Verification items for the finished model (mm, model axes). A direction names the side the tool comes from. Coordinates: 2 decimals unless noted, no trailing zeros. Loops run counter-clockwise (first coordinate to the right, second up) from the corner with the lowest first, then second, coordinate; pieces in that order, holes last. Notation, with made-up numbers: (-35, 36) - (-8, 36) arc R21 ccw to (-8, 45) - close; hole circle Ø7 at (-33, -39.5). An arc over 180 degrees is marked (long way). One line per item, written item: value. Start each with the question number.
(1) Thickness scan on probe 1 along Y at (x, z) = (-50, 6); probe 2 along Y at (x, z) = (11, 66); probe 3 along Y at (x, z) = (-3.5, 134.5). Record the ranges inside material, lowest first. Write a range as [from, to].
(2) Gauge pin test, flat ends, axial feed: P1, Ø12, axis at y = 24.5, z = 31, coming from the -X side; P2, Ø5, axis at x = -6, y = 2.5, coming from the +Z side; P3, Ø6, axis at x = 33, y = -17.5, coming from the -Z side; P4, Ø4, axis at x = -12, z = 26, coming from the -Y side. Record the tip position at first contact, or that the pin passes through.
(3) Section check B-B (y = -20). Record the boundary of the cut face in (x, z).
(4) Draft check along Z on faces 4 (the face through (-58, -32, 10)), 5 (the face through (0, -18, 70)), 6 (the face through (32, 25, 21)). Enter one of: +Z half, -Z half, draft (parallel to the pull), parting line (faces both ways), or undercut.
(5) Set-up check for faces 1 (the face through (-6.503, -29.126, 149.287)), 2 (the face through (30, 26, 72)), 3 (the face through (4, 15, 129)): record each of +Z, -Z, +X, -X, +Y, -Y from which the full face is reachable in a straight line by a thin tool's end or side.
(6) Section check C-C (z = 132). Record the boundary of the cut face in (x, y), plus the area to 3 significant figures.
(7) Section check A-A (x = -50). Record the boundary of the cut face in (y, z).
(8) Section check D-D (x = 0). Record the boundary of the cut face in (y, z), plus the area to 3 significant figures.
```python
from build123d import *

# Parameters (mm, degrees)
Y_KSEKLIK_EKSTR_ZYON1_DEPTH = 20
Y_KSEKLIK_EKSTR_ZYON2_DEPTH = 15
Y_KSEKLIK_EKSTR_ZYON3_START = 3
IZIM3_R                     = 30
Y_KSEKLIK_EKSTR_ZYON3_DEPTH = 3
IZIM4_R                     = 20
Y_KSEKLIK_EKSTR_ZYON4_DEPTH = 3
IZIM5_R                     = 10
KES_EKSTR_ZYON1_DEPTH       = 169.534862862
AYNALAMA1_START             = -33
AYNALAMA1_OUTLINE_R         = 10
AYNALAMA1_DEPTH             = 15
AYNALAMA1_START_2           = -36
AYNALAMA1_2_OUTLINE_R       = 30
AYNALAMA1_2_OUTLINE_R_2     = 10
AYNALAMA1_2_DEPTH           = 3
AYNALAMA1_START_3           = -18
AYNALAMA1_3_OUTLINE_R       = 20
AYNALAMA1_3_OUTLINE_R_2     = 10
AYNALAMA1_3_DEPTH           = 3
IZIM6_R                     = 5.25
KES_EKSTR_ZYON2_DEPTH       = 148.634684272
RADYUS1_R                   = 5


# Read off the part's stored shape, not the designer's step: Aynalama1
with BuildPart() as part:
    # izim1 → Y_kseklik-Ekstr_zyon1 (new body)
    with BuildSketch(Plane.XY):
        with BuildLine():
            Line((-55, 33), (55, 33))
            ThreePointArc((55, 33), (58.535533906, 31.535533906), (60, 28))
            Line((60, 28), (60, -28))
            ThreePointArc((60, -28), (58.535533906, -31.535533906), (55, -33))
            Line((55, -33), (-55, -33))
            ThreePointArc((-55, -33), (-58.535533906, -31.535533906), (-60, -28))
            Line((-60, -28), (-60, 28))
            ThreePointArc((-60, 28), (-58.535533906, 31.535533906), (-55, 33))
        make_face()
    extrude(amount=Y_KSEKLIK_EKSTR_ZYON1_DEPTH)

    # izim2 → Y_kseklik-Ekstr_zyon2 (add)
    with BuildSketch(Plane(origin=(0, 33, 0), x_dir=(1, 0, 0), z_dir=(0, 1, 0))):
        with BuildLine():
            Line((-30, -20), (30, -20))
            Line((30, -20), (30, -120))
            ThreePointArc((30, -120), (0, -150), (-30, -120))
            Line((-30, -120), (-30, -20))
        make_face()
    extrude(amount=-Y_KSEKLIK_EKSTR_ZYON2_DEPTH)

    # izim3 → Y_kseklik-Ekstr_zyon3 (add)
    with BuildSketch(Plane(origin=(0, 33, 0), x_dir=(1, 0, 0), z_dir=(0, 1, 0)).offset(Y_KSEKLIK_EKSTR_ZYON3_START)):
        with Locations(Location((0, -120, 0), (0, 0, 270))):
            Circle(IZIM3_R)
    extrude(amount=-Y_KSEKLIK_EKSTR_ZYON3_DEPTH)

    # izim4 → Y_kseklik-Ekstr_zyon4 (add)
    with BuildSketch(Plane(origin=(0, 18, 0), x_dir=(-1, 0, 0), z_dir=(0, -1, 0))):
        with Locations(Location((0, -120, 0), (0, 0, 270))):
            Circle(IZIM4_R)
    extrude(amount=Y_KSEKLIK_EKSTR_ZYON4_DEPTH)

    # izim5 → Kes-Ekstr_zyon1 (cut, through all)
    with BuildSketch(Plane.XZ.offset(-15)):
        with Locations(Location((0, 118.867910889, 0), (0, 0, 270))):
            Circle(IZIM5_R)
    extrude(amount=-KES_EKSTR_ZYON1_DEPTH, mode=Mode.SUBTRACT)

    # Aynalama1 outline → Aynalama1 (add)
    with BuildSketch(Plane(origin=(0, 0, 0), x_dir=(1, 0, 0), z_dir=(0, 1, 0)).offset(AYNALAMA1_START)):
        with BuildLine():
            Line((-30, -20), (-30, -120))
            ThreePointArc((-30, -120), (0, -150), (30, -120))
            Line((30, -120), (30, -20))
            Line((30, -20), (-30, -20))
        make_face()
        with Locations((0, -118.867910889)):
            Circle(AYNALAMA1_OUTLINE_R, mode=Mode.SUBTRACT)
    extrude(amount=AYNALAMA1_DEPTH)

    # Aynalama1 2 outline → Aynalama1 2 (add)
    with BuildSketch(Plane(origin=(0, 0, 0), x_dir=(1, 0, 0), z_dir=(0, 1, 0)).offset(AYNALAMA1_START_2)):
        with Locations((0, -120)):
            Circle(AYNALAMA1_2_OUTLINE_R)
        with Locations((0, -118.867910889)):
            Circle(AYNALAMA1_2_OUTLINE_R_2, mode=Mode.SUBTRACT)
    extrude(amount=AYNALAMA1_2_DEPTH)

    # Aynalama1 3 outline → Aynalama1 3 (add)
    with BuildSketch(Plane(origin=(0, 0, 0), x_dir=(1, 0, 0), z_dir=(0, 1, 0)).offset(AYNALAMA1_START_3)):
        with Locations((0, -120)):
            Circle(AYNALAMA1_3_OUTLINE_R)
        with Locations((0, -118.867910889)):
            Circle(AYNALAMA1_3_OUTLINE_R_2, mode=Mode.SUBTRACT)
    extrude(amount=AYNALAMA1_3_DEPTH)

    # izim6 → Kes-Ekstr_zyon2 (cut, through all)
    with BuildSketch(Plane.XY.offset(20)):
        with Locations((-50, 20)):
            Circle(IZIM6_R)
        with Locations((-50, -20)):
            Circle(IZIM6_R)
        with Locations(Location((50, -20, 0), (0, 0, 180))):
            Circle(IZIM6_R)
        with Locations(Location((50, 20, 0), (0, 0, 180))):
            Circle(IZIM6_R)
    extrude(amount=-KES_EKSTR_ZYON2_DEPTH, mode=Mode.SUBTRACT)

    # Radyus1
    radyus1_edges = [part.edges().sort_by_distance(p)[0] for p in [
        (-30, 25.5, 20),
        (30, 25.5, 20),
        (-30, -25.5, 20),
        (30, -25.5, 20),
    ]]
    fillet(radyus1_edges, radius=RADYUS1_R)


solid = part.part
```
Responses:
1. probe 1: y = [-33, -25.25], [-14.75, 14.75], [25.25, 33]
1. probe 2: y = [-33, -18], [18, 33]
1. probe 3: y = [-36, -15], [15, 36]
2. P1: stops at x = -30
2. P2: stops at z = 20
2. P3: stops at z = 0
2. P4: stops at y = -33
3. outline: (-60, 0) - (-55.25, 0) - (-55.25, 20) - (-60, 20) - close; (-44.75, 0) - (44.75, 0) - (44.75, 20) - (35, 20) arc R5 cw to (30, 25) - (30, 120) arc R30 ccw to (-30, 120) - (-30, 25) arc R5 cw to (-35, 20) - (-44.75, 20) - close; (55.25, 0) - (60, 0) - (60, 20) - (55.25, 20) - close; hole circle Ø20 at (0, 118.87)
4. face 4: draft
4. face 5: undercut
4. face 6: +Z half
5. face 1: -Y
5. face 2: +Z, +X, +Y, -Y
5. face 3: +Z, +X, -X
6. outline: (-27.5, -36) - (27.5, -36) - (27.5, -18) - (16, -18) - (16, -15) - (-16, -15) - (-16, -18) - (-27.5, -18) - close; (-27.5, 18) - (-16, 18) - (-16, 15) - (16, 15) - (16, 18) - (27.5, 18) - (27.5, 36) - (-27.5, 36) - close
6. area: 2,170 mm²
7. outline: (-33, 0) - (-25.25, 0) - (-25.25, 20) - (-33, 20) - close; (-14.75, 0) - (14.75, 0) - (14.75, 20) - (-14.75, 20) - close; (25.25, 0) - (33, 0) - (33, 20) - (25.25, 20) - close
8. outline: (-36, 90) - (-33, 90) - (-33, 0) - (33, 0) - (33, 90) - (36, 90) - (36, 108.87) - (15, 108.87) - (15, 100) - (18, 100) - (18, 20) - (-18, 20) - (-18, 100) - (-15, 100) - (-15, 108.87) - (-36, 108.87) - close; (-36, 128.87) - (-15, 128.87) - (-15, 140) - (-18, 140) - (-18, 150) - (-36, 150) - close; (15, 128.87) - (36, 128.87) - (36, 150) - (18, 150) - (18, 140) - (15, 140) - close
8. area: 4,980 mm²
